Work out the finished part from the listing and answer in its coordinate system (mm). Face numbers are marked on the shaded views. A direction names the side the tool comes from. Round coordinates to 2 decimals unless told otherwise and drop trailing zeros. Loops run counter-clockwise (first coordinate to the right, second up) from the corner with the lowest first, then second, coordinate; pieces in that order, holes last.
```python
from build123d import *

# Parameters (mm, degrees)
ESQUISSE1_R             = 6
BOSS_EXTRU_1_DEPTH      = 190
ESQUISSE2_R             = 7
BOSS_EXTRU_2_DEPTH      = 35
ESQUISSE3_R             = 3
ENL_V_MAT_EXTRU_1_DEPTH = 20
ESQUISSE4_W             = 10.048379513
ESQUISSE4_H             = 5
ENL_V_MAT_EXTRU_2_DEPTH = 29


with BuildPart() as part:
    # Esquisse1 → Boss.-Extru.1 (new body)
    with BuildSketch(Plane.XY):
        Circle(ESQUISSE1_R)
    extrude(amount=BOSS_EXTRU_1_DEPTH)

    # Esquisse2 → Boss.-Extru.2 (add)
    with BuildSketch(Plane.XY.offset(190)):
        Circle(ESQUISSE2_R)
    extrude(amount=BOSS_EXTRU_2_DEPTH)

    # Esquisse3 → Enlèv. mat.-Extru.1 (cut)
    with BuildSketch(Plane(origin=(0, 0, 0), x_dir=(-1, 0, 0), z_dir=(0, 0, -1))):
        Circle(ESQUISSE3_R)
    extrude(amount=-ENL_V_MAT_EXTRU_1_DEPTH, mode=Mode.SUBTRACT)

    # Esquisse4 → Enlèv. mat.-Extru.2 (cut)
    with BuildSketch(Plane.XY.offset(225)):
        with Locations((0.381691631, 8)):
            Rectangle(ESQUISSE4_W, ESQUISSE4_H)
    extrude(amount=-ENL_V_MAT_EXTRU_2_DEPTH, mode=Mode.SUBTRACT)


solid = part.part
```
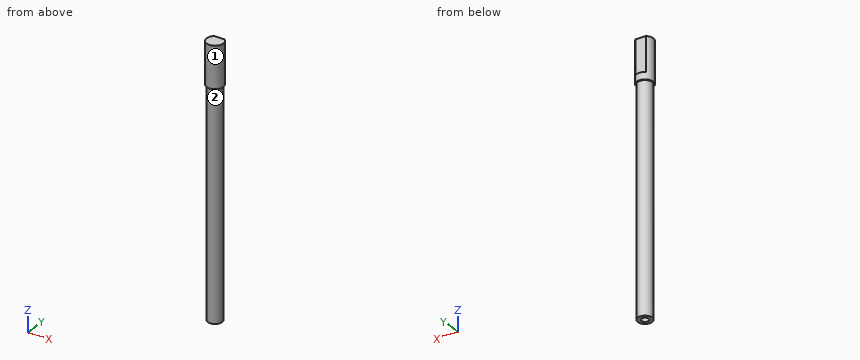
1. Consider probe 1 along Y at (x, z) = (0, 8); probe 2 along Z at (x, y) = (5, -4.5); probe 3 along X at (y, z) = (-0.25, 66.5). Determine where each line is inside the solid, lowest interval first.
Answer key:
probe 1: y = -6 to -3, 3 to 6
probe 2: z = 190 to 225
probe 3: x = -5.99 to 5.99
2. Find section B-B (x = 0). Write down the section's boundary in (y, z), then the cut area to 3 significant figures.
Answer key:
outline: (-7, 190) - (-6, 190) - (-6, 0) - (-3, 0) - (-3, 20) - (3, 20) - (3, 0) - (6, 0) - (6, 190) - (7, 190) - (7, 196) - (5.5, 196) - (5.5, 225) - (-7, 225) - close
area: 2,610 mm2
3. Which of the six approach directions +Z, -Z, +X, -X, +Y, -Y give full straight-line access (tool end or side, diameter ignored) to the marked faces 1 and 2?
Answer key:
face 1: +Z, -Z
face 2: -Z
4. Given pin 1 (1 mm diameter, centred on y = -2.5, z = 182.5, fed in from +X); pin 2 (2 mm diameter, centred on x = -4.5, z = 101, fed in from -Y); pin 3 (7 mm diameter, centred on x = -1, z = 203.5, fed in from +Y), each flat-ended and moving along its own axis, determine where each tip first touches the part or whether it passes through.
Answer key:
pin 1: stops at x = 5.66
pin 2: stops at y = -4.87
pin 3: stops at y = 5.5
5. Find section A-A (y = 0). Write down the section's boundary in (x, z), then the cut area to 3 significant figures.
Answer key:
outline: (-7, 190) - (-6, 190) - (-6, 0) - (-3, 0) - (-3, 20) - (3, 20) - (3, 0) - (6, 0) - (6, 190) - (7, 190) - (7, 225) - (-7, 225) - close
area: 2,650 mm2
6. Find section C-C (z = 126). Write down the section's boundary in (x, y).
Answer key:
outline: circle Ø12 at (0, 0)
